from build123d import *

# Parameters (mm, degrees)
F1_DEPTH  = 25.4
F4_W      = 12.7
F4_H      = 5.478115
F5_DEPTH  = 12.7
F3_R      = 2.658023
F6_DEPTH  = 25.4
F7_R      = 2.706584
F8_DEPTH  = 25.4
F9_R      = 3.81
F11_DEPTH = 7.62
F10_R     = 3.81
F12_DEPTH = 7.62


with BuildPart() as f1:
    # F0 (on Top) → F1 (new body)
    with BuildSketch(Plane.XY):
        with BuildLine():
            ThreePointArc((0, 6.35), (1.859872, 1.859872), (6.35, 0))
            Line((6.35, 0), (31.75, 0))
            ThreePointArc((31.75, 0), (36.240128, 1.859872), (38.1, 6.35))
            Line((38.1, 6.35), (38.1, 31.75))
            ThreePointArc((38.1, 31.75), (36.240128, 36.240128), (31.75, 38.1))
            Line((31.75, 38.1), (6.35, 38.1))
            ThreePointArc((6.35, 38.1), (1.859872, 36.240128), (0, 31.75))
            Line((0, 31.75), (0, 6.35))
        make_face()
    extrude(amount=F1_DEPTH)

    # F4 (on face) → F5 (join)
    with BuildSketch(Plane.XY.offset(25.4)):
        with Locations((19.05, 22.330752)):
            Rectangle(F4_W, F4_H)
    extrude(amount=F5_DEPTH)

    # F3 (on face) → F6 (cut)
    with BuildSketch(Plane.XY.offset(25.4)):
        with Locations((19.05, 19.05)):
            Circle(F3_R)
    extrude(amount=-F6_DEPTH, mode=Mode.SUBTRACT)

    # F7 (on face) → F8 (cut)
    with BuildSketch(Plane.XY.offset(38.1)):
        with Locations((19.05, 19.05)):
            Circle(F7_R)
    extrude(amount=-F8_DEPTH, mode=Mode.SUBTRACT)

    # F9 (on face) → F11 (join)
    with BuildSketch(Plane.XZ):
        with Locations((19.05, 16.51)):
            Circle(F9_R)
    extrude(amount=F11_DEPTH)

    # F10 (on face) → F12 (join)
    with BuildSketch(Plane(origin=(0, 38.1, 0), x_dir=(-1, 0, 0), z_dir=(0, 1, 0))):
        with Locations((-19.05, 16.51)):
            Circle(F10_R)
    extrude(amount=F12_DEPTH)


solid = f1.part
Geometry check sheet. Reference: the model listing, model coordinates, mm. A direction names the side the tool comes from. Coordinates: 2 decimals unless noted, no trailing zeros. Order: outer loops, then holes, each group sorted by start corner. A loop starts at its lowest first (then second) coordinate and runs counter-clockwise, first axis right, second up. Notation, with made-up numbers: (5, 40) - (22, 40) arc R16 cw to (22, 70) - close; hole circle Ø10 at (-20, -21.5). An arc over 180 degrees is marked (long way). One line per item, written item: value.
(1) Sectioned sample at C-C (y = 23.5). Enter the section's corners in (x, z).
Data:
outline: (0, 0) - (38.1, 0) - (38.1, 25.4) - (25.4, 25.4) - (25.4, 38.1) - (12.7, 38.1) - (12.7, 25.4) - (0, 25.4) - close
(2) Depth check by flat-ended pin: pin 1 Ø8 at (x, z) = (15, 24.5) entering from -Y; pin 2 Ø6 at (x, y) = (19.05, 19.05) entering from +Z; pin 3 Ø1.1 at (x, z) = (23.5, 32.5) entering from -Y; pin 4 Ø4.5 at (x, y) = (19.5, 18.5) entering from +Z. Enter the tip coordinate at first touch or a pass-through.
Data:
pin 1: stops at y = 0
pin 2: stops at z = 38.1
pin 3: stops at y = 19.59
pin 4: stops at z = 25.4
(3) Access from +Z, -Z, +X, -X, +Y, -Y to the whole of each face (thin tool, end or side, straight path). Record for faces 1 (the face through (18.554, -3.757, 20.288)), 2 (the face through (17, 41.86, 19.72)), 3 (the face through (25.4, 22, 32)), 4 (the face through (23, 19, 0)), 5 (the face through (15, 19.592, 32)).
Data:
face 1: -Y
face 2: +Y
face 3: +Z, +X, +Y, -Y
face 4: -Z, +X, -X, +Y, -Y
face 5: +Z, +X, -X, -Y
(4) Release check for a two-part mould opening along Y. For faces 6 (the face through (36.19, 1.81, 12.52)), 7 (the face through (18.474, 16.455, 6.439)), 8 (the face through (12.7, 22, 32)) record: +Y half, -Y half, draft (parallel to the pull), parting line (faces both ways), or undercut.
Data:
face 6: -Y half
face 7: undercut
face 8: draft
(5) Thickness scan on probe 1 along Y at (x, z) = (19, 23); probe 2 along X at (y, z) = (19, 9). Record the ranges inside material, lowest first. Write a range as from..to.
Data:
probe 1: y = 0..16.34, 21.76..38.1
probe 2: x = 0..16.39, 21.71..38.1
(6) Sectioned sample at B-B (x = 19.05). Enter the section's corners in (y, z).
Data:
outline: (-7.62, 12.7) - (0, 12.7) - (0, 0) - (16.39, 0) - (16.39, 12.7) - (16.34, 12.7) - (16.34, 25.4) - (0, 25.4) - (0, 20.32) - (-7.62, 20.32) - close; (21.71, 0) - (38.1, 0) - (38.1, 12.7) - (45.72, 12.7) - (45.72, 20.32) - (38.1, 20.32) - (38.1, 25.4) - (25.07, 25.4) - (25.07, 38.1) - (21.76, 38.1) - (21.76, 12.7) - (21.71, 12.7) - close
(7) Sectioned sample at A-A (z = 11). Enter the section's corners in (x, y).
Data:
outline: (0, 6.35) arc R6.35 ccw to (6.35, 0) - (31.75, 0) arc R6.35 ccw to (38.1, 6.35) - (38.1, 31.75) arc R6.35 ccw to (31.75, 38.1) - (6.35, 38.1) arc R6.35 ccw to (0, 31.75) - close; hole circle Ø5.32 at (19.05, 19.05)
(8) Sectioned sample at D-D (z = 16.51). Enter the section's corners in (x, y), and give its area (3 significant figures).
Data:
outline: (0, 6.35) arc R6.35 ccw to (6.35, 0) - (15.24, 0) - (15.24, -7.62) - (22.86, -7.62) - (22.86, 0) - (31.75, 0) arc R6.35 ccw to (38.1, 6.35) - (38.1, 31.75) arc R6.35 ccw to (31.75, 38.1) - (22.86, 38.1) - (22.86, 45.72) - (15.24, 45.72) - (15.24, 38.1) - (6.35, 38.1) arc R6.35 ccw to (0, 31.75) - close; hole circle Ø5.41 at (19.05, 19.05)
area: 1,510 mm^2
